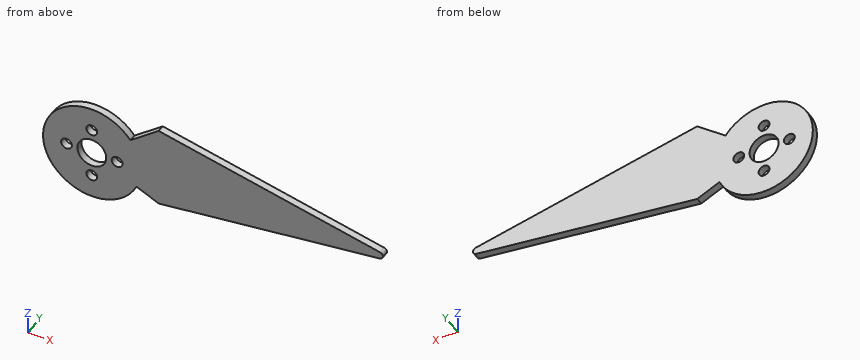
from build123d import *

# Parameters (mm, degrees)
BRIDA_BASE1_DEPTH     = 2
CROQUIS12_R           = 4
CORTAR_EXTRUIR1_DEPTH = 2
CROQUIS13_R           = 1.5
CORTAR_EXTRUIR2_DEPTH = 2
MATRIZC1_COUNT        = 4


# Sheet-metal steps are written as plain solids
with BuildPart() as part:
    # Croquis7 → Brida base1 (new body)
    with BuildSketch(Plane(origin=(0, 0, 0), x_dir=(1, 0, 0), z_dir=(0, 1, 0))):
        with BuildLine():
            Line((10.659249118, -8.284752463), (18.5, -14.378866547))
            Line((18.5, -14.378866547), (79.710147148, -1.70472983))
            ThreePointArc((79.710147148, -1.70472983), (80.506688025, -0.68807512), (79.636333375, 0.266150717))
            Line((79.636333375, 0.266150717), (18.5, 8.215724958))
            Line((18.5, 8.215724958), (12.337716326, 5.480645126))
            ThreePointArc((12.337716326, 5.480645126), (-13.400994276, 1.634034128), (10.659249118, -8.284752463))
        make_face()
    extrude(amount=-BRIDA_BASE1_DEPTH)

    # Croquis12 → Cortar-Extruir1 (cut)
    with BuildSketch(Plane(origin=(0, 0, 0), x_dir=(1, 0, 0), z_dir=(0, 1, 0))):
        with Locations(Location((0, 0, 0), (0, 0, 270))):
            Circle(CROQUIS12_R)
    extrude(amount=-CORTAR_EXTRUIR1_DEPTH, mode=Mode.SUBTRACT)

    # Croquis13 → Cortar-Extruir2 (cut)
    with BuildSketch(Plane(origin=(0, 0, 0), x_dir=(1, 0, 0), z_dir=(0, 1, 0))):
        with Locations(Location((0, 7, 0), (0, 0, 270))):
            Circle(CROQUIS13_R)
    cortar_extruir2 = extrude(amount=-CORTAR_EXTRUIR2_DEPTH, mode=Mode.SUBTRACT)

    # MatrizC1: Cortar-Extruir2 ×4 about axis
    matrizc1_axis = Axis((0, 0, 0), (0, 1, 0))
    for i in range(1, MATRIZC1_COUNT):
        add(cortar_extruir2.rotate(matrizc1_axis, i * 360 / MATRIZC1_COUNT), mode=Mode.SUBTRACT)


solid = part.part
Read the model definition and answer for the solid it produces. Units are mm, in the model's axes. Coordinates: 2 decimals unless noted, no trailing zeros. Loops run counter-clockwise (first coordinate to the right, second up) from the corner with the lowest first, then second, coordinate; pieces in that order, holes last. Notation, with made-up numbers: (-1, 77.25) -> (4, 77.25) arc R33 ccw to (4, 112.25) -> close; hole circle Ø6 at (22.25, 46.25). An arc over 180 degrees is marked (long way). Write item = value, one per line. Start each with the question number.
1) The part is cut by section C-C, the plane z = 7. Determine the outline of the cut face in (x, y), plus the area to 3 significant figures.
2) The part is cut by section A-A, the plane x = 0. Determine the outline of the cut face in (y, z).
3) Find the intervals of material crossed by L1, parallel to Z at x = -1, y = -0.4; L2, parallel to X at y = -0.2, z = -10.5; L3, parallel to Z at x = -7.5, y = -0.35, in increasing order. Write a range as from..to.
4) The part is cut by section D-D, the plane z = -7. Determine the outline of the cut face in (x, y).
5) The part is cut by section B-B, the plane y = -0.8. Determine the outline of the cut face in (x, z), plus the area to 3 significant figures.
Result:
q1.outline = (-11.54, -2) -> (-1.5, -2) -> (-1.5, 0) -> (-11.54, 0) -> close; (1.5, -2) -> (54.14, -2) -> (54.14, 0) -> (1.5, 0) -> close
q1.area = 125 mm²
q2.outline = (-2, -13.5) -> (0, -13.5) -> (0, -8.5) -> (-2, -8.5) -> close; (-2, -5.5) -> (0, -5.5) -> (0, -4) -> (-2, -4) -> close; (-2, 4) -> (0, 4) -> (0, 5.5) -> (-2, 5.5) -> close; (-2, 8.5) -> (0, 8.5) -> (0, 13.5) -> (-2, 13.5) -> close
q3.L1 = -13.46..-8.12, -5.88..-3.87, 3.87..5.88, 8.12..13.46
q3.L2 = -8.49..8.49
q3.L3 = -11.23..-1.41, 1.41..11.23
q4.outline = (-11.54, -2) -> (-1.5, -2) -> (-1.5, 0) -> (-11.54, 0) -> close; (1.5, -2) -> (11.54, -2) -> (11.54, 0) -> (1.5, 0) -> close; (15.76, -2) -> (27.85, -2) -> (27.85, 0) -> (15.76, 0) -> close
q5.outline = (10.66, 8.28) arc R13.5 ccw (long way) to (12.34, -5.48) -> (18.5, -8.22) -> (79.64, -0.27) arc R1 ccw to (79.71, 1.7) -> (18.5, 14.38) -> close; hole circle Ø3 at (-7, 0); hole circle Ø8 at (0, 0); hole circle Ø3 at (0, -7); hole circle Ø3 at (0, 7); hole circle Ø3 at (7, 0)
q5.area = 1,360 mm²
